from build123d import *

# Parameters (mm, degrees)
SKETCH1_W           = 101.6
SKETCH1_H           = 50.8
BOSS_EXTRUDE1_DEPTH = 5.9436
SKETCH2_R           = 4.7625
CUT_EXTRUDE1_DEPTH  = 6.9436
SKETCH3_W           = 5.94334
SKETCH3_H           = 12.7
BOSS_EXTRUDE2_DEPTH = 5.9436
CUT_EXTRUDE2_DEPTH  = 6.9436


with BuildPart() as part:
    # Sketch1 → Boss-Extrude1 (new body)
    with BuildSketch(Plane.XY):
        with Locations((50.8, 25.4)):
            Rectangle(SKETCH1_W, SKETCH1_H)
    extrude(amount=BOSS_EXTRUDE1_DEPTH)

    # Sketch2 → Cut-Extrude1 (cut, through all)
    with BuildSketch(Plane.XY.offset(5.9436)):
        with Locations((50.8, 25.4)):
            Circle(SKETCH2_R)
    extrude(amount=-CUT_EXTRUDE1_DEPTH, mode=Mode.SUBTRACT)

    # Sketch3 → Boss-Extrude2 (add)
    with BuildSketch(Plane(origin=(0, 0, 0), x_dir=(-1, 0, 0), z_dir=(0, 0, -1))):
        with Locations((2.97167, 25.492131347)):
            Rectangle(SKETCH3_W, SKETCH3_H)
    extrude(amount=-BOSS_EXTRUDE2_DEPTH)

    # Sketch5 → Cut-Extrude2 (cut, through all)
    with BuildSketch(Plane(origin=(0, 0, 0), x_dir=(-1, 0, 0), z_dir=(0, 0, -1))):
        Polygon((0, 41.798931347), (-4.60401, 41.798931347), (-4.60401, 40.097131347), (-6.98526, 40.097131347), (-6.98526, 41.798931347), (-9.52526, 41.798931347), (-9.52526, 44.745331347), (-6.98526, 44.745331347), (-6.98526, 46.447131347), (-4.60401, 46.447131347), (-4.60401, 44.745331347), (0, 44.745331347), align=None)
        Polygon((-4.60401, 4.537131347), (-4.60401, 6.238931347), (0, 6.238931347), (0, 9.185331347), (-4.60401, 9.185331347), (-4.60401, 10.887131347), (-6.98526, 10.887131347), (-6.98526, 9.185331347), (-9.52526, 9.185331347), (-9.52526, 6.238931347), (-6.98526, 6.238931347), (-6.98526, 4.537131347), align=None)
    extrude(amount=-CUT_EXTRUDE2_DEPTH, mode=Mode.SUBTRACT)


solid = part.part
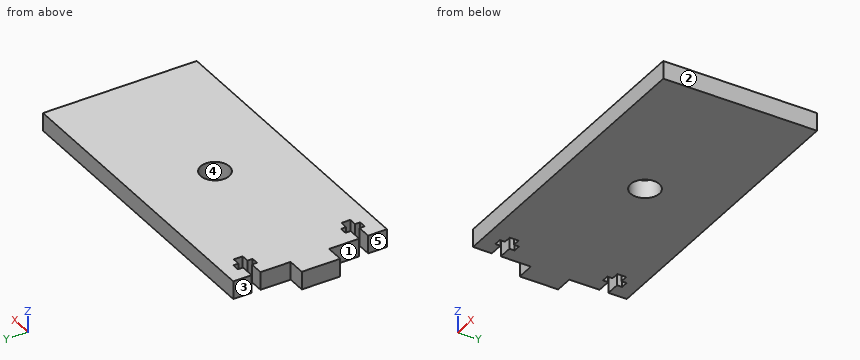
Verification items for the finished model (mm, model axes). Face numbers are marked on the shaded views. A direction names the side the tool comes from. Coordinates: 2 decimals unless noted, no trailing zeros. Order: outer loops, then holes, each group sorted by start corner. A loop starts at its lowest first (then second) coordinate and runs counter-clockwise, first axis right, second up.
Item 1: Access from +Z, -Z, +X, -X, +Y, -Y to the whole of each face (thin tool, end or side, straight path). Record for the marked faces 1, 2 and 3.
Filled in:
face 1: +Z, -Z, -X, -Y
face 2: +Z, -Z, +X, +Y, -Y
face 3: +Z, -Z, -X, +Y
Item 2: Material ranges on L1, parallel to Y at x = 0.5, z = 3.85; L2, parallel to Y at x = 50.8, z = 2.3; L3, parallel to X at y = 22, z = 2.65, recorded low to high.
Filled in:
L1: y = 0 to 6.24, 9.19 to 41.8, 44.75 to 50.8
L2: y = 0 to 20.64, 30.16 to 50.8
L3: x = -5.94 to 47.47, 54.13 to 101.6
Item 3: Depth check by flat-ended pin: pin 1 (0.9 mm diameter, centred on y = 41, z = 4.5, fed in from -X); pin 2 (3 mm diameter, centred on x = -3, z = 2.5, fed in from -Y). Enter the tip coordinate at first touch or a pass-through.
Filled in:
pin 1: stops at x = 0
pin 2: stops at y = 19.14
Item 4: Section check B-B, the plane x = 50.8. Enter the section's corners in (y, z).
Filled in:
outline: (0, 0) - (20.64, 0) - (20.64, 5.94) - (0, 5.94) - close; (30.16, 0) - (50.8, 0) - (50.8, 5.94) - (30.16, 5.94) - close
Item 5: Release check for a two-part mould opening along Y. For the marked faces 4 and 5 record: +Y half, -Y half, draft (parallel to the pull), parting line (faces both ways), or undercut.
Filled in:
face 4: undercut
face 5: draft
Item 6: Section check C-C, the plane y = 25.4. Enter the section's corners in (x, z), then the cut area to 3 significant figures.
Filled in:
outline: (-5.94, 0) - (46.04, 0) - (46.04, 5.94) - (-5.94, 5.94) - close; (55.56, 0) - (101.6, 0) - (101.6, 5.94) - (55.56, 5.94) - close
area: 583 mm2
Item 7: Section check A-A, the plane x = 3. Enter the section's corners in (y, z), then the cut area to 3 significant figures.
Filled in:
outline: (0, 0) - (6.24, 0) - (6.24, 5.94) - (0, 5.94) - close; (9.19, 0) - (41.8, 0) - (41.8, 5.94) - (9.19, 5.94) - close; (44.75, 0) - (50.8, 0) - (50.8, 5.94) - (44.75, 5.94) - close
area: 267 mm2
